Autodesk Inventor part; units mm, degrees
ref_plane "YZ Plane" through (0, 0, 0) normal (1, 0, 0) x (0, 1, 0)
ref_plane "XZ Plane" through (0, 0, 0) normal (0, 1, 0) x (-1, 0, 0)
ref_plane "XY Plane" through (0, 0, 0) normal (0, 0, 1) x (1, 0, 0)
sketch "Boceto1" plane through (0, 0, 0) normal (0, 1, 0) x (-1, 0, 0)
  line L0 (-13, -23) -> (13, -23)
  line L1 (13, -23) -> (13, 23)
  line L2 (13, 23) -> (-13, 23)
  line L3 (-13, 23) -> (-13, -23)
  line L4 (-13, -23) -> (13, 23) construction
  line L5 (13, -23) -> (-13, 23) construction
  line L6 (-14.5, -25) -> (14.5, -25)
  line L7 (14.5, -25) -> (14.5, 25)
  line L8 (14.5, 25) -> (-14.5, 25)
  line L9 (-14.5, 25) -> (-14.5, -25)
  line L10 (-14.5, -25) -> (14.5, 25) construction
  line L11 (14.5, -25) -> (-14.5, 25) construction
  point P0 (0, 0)
  dimension "d0" = 46
  dimension "d1" = 26
  dimension "d2" = 2
  dimension "d3" = 1.5
extrude "Extrusión1" add sketch "Boceto1" along normal blind 19.5 contours L3 L2 L1 L0 | L9 L8 L7 L6
sketch "Boceto2" plane through (0, 19.5, 0) normal (0, 1, 0) x (1, 0, 0)
  line L0 (-13, -23) -> (13, -23)
  line L1 (13, -23) -> (13, 23)
  line L2 (13, 23) -> (-13, 23)
  line L3 (-13, 23) -> (-13, -23)
  point P0 (0, 0)
extrude "Extrusión2" cut sketch "Boceto2" against normal blind 16.25
sketch "Boceto3" plane through (-14.5, 0, 25) normal (0, 0, 1) x (1, 0, 0)
  line L0 (29, 19.5) -> (0, 19.5)
  line L1 (13.0274, 19.5) -> (13.0274, 8.5)
  line L2 (17.0274, 19.5) -> (17.0274, 8.5)
  line L3 (3.0274, 19.5) -> (3.0274, 8.5)
  line L4 (27.0274, 19.5) -> (27.0274, 8.5)
  arc A0 (3.0274, 8.5) -> (13.0274, 8.5) centre (8.0274, 8.5) ccw
  arc A1 (17.0274, 8.5) -> (27.0274, 8.5) centre (22.0274, 8.5) ccw
  point P0 (14.5, 0)
  dimension "d8" = 11
  dimension "d10" = 10
  dimension "d11" = 10
  dimension "d12" = 4
  dimension "d13" = 11
  dimension "d14" = 11
  dimension "d15" = 11
extrude "Extrusión3" cut sketch "Boceto3" against normal blind 17
sketch "Boceto4" plane through (-14.5, 0, -25) normal (-1, 0, 0) x (0, 0, 1)
  line L0 (48, 19.5) -> (2, 19.5)
  arc A0 (10.16, 19.5) -> (39.84, 19.5) centre (25, 30.7495) ccw
  line L1 (0, 0) -> (0, 19.5)
  line L2 (50, 0) -> (50, 19.5)
  point P0 (25, 0)
  dimension "d18" = 10.16
  dimension "d19" = 10.16
extrude "Extrusión4" cut sketch "Boceto4" against normal blind 17
sketch "Boceto5" plane through (14.5, 0, 25) normal (1, 0, 0) x (0, 0, -1)
  line L0 (48, 19.5) -> (2, 19.5)
  arc A0 (10.16, 19.5) -> (39.84, 19.5) centre (25, 35.1546) ccw
  line L1 (50, 0) -> (50, 19.5)
  line L2 (0, 0) -> (0, 19.5)
  point P0 (25, 0)
  dimension "d22" = 10.16
  dimension "d23" = 10.16
extrude "Extrusión5" cut sketch "Boceto5" against normal blind 17
fillet "Empalme1" radius 2 8 edges at (13.75, 19.5, -14.84) (13.75, 19.5, 14.84) (13.5137, 19.5, 25) (-13.75, 19.5, -14.84) (-13.75, 19.5, 14.84) (-12.9863, 19.5, 25) (0.5274, 19.5, 25) (0, 19.5, -25)
properties part number "CASE batería"
The model under review builds one solid part; all positions refer to its coordinate system, in mm. A direction names the side the tool comes from. Give positions to 0.01 mm unless a question says otherwise; leave off trailing zeros. Write each loop counter-clockwise with the first axis right and the second up, starting at its lowest first coordinate (ties: lowest second). Pieces come first, ordered by that corner, then holes. Notation, with made-up numbers: (64.5, 1) - (94.5, 1) arc R21 cw to (94.5, 23) - close; hole circle Ø9 at (44.25, 2.25). An arc over 180 degrees is marked (long way). Answer in a Markdown table with one row per item. Add a question column.
1. We need section B-B on y = 18.25. Write out the cut boundary in (x, z), then the cut area to 3 significant figures.
2. Draft analysis for pull direction X (two halves, no side actions). For faces 6 (the flat face through (-11.473, 14, 24)), 7 (the flat face through (14, 19.5, 19)), state which applies: +X half, -X half, draft (parallel to the pull), parting line (faces both ways), or undercut.
3. Wall thickness on line 1 along X through (y, z) = (8, 22.5); line 2 along Z through (x, y) = (-3.5, 3.5); line 3 along Y through (x, z) = (2.75, -1): over which ranges is each line inside the solid? List them lowest first. Write a range as [from, to].
4. Tool access review of faces 1 (the flat face through (13, 10, 0)), 2 (the cylindrical face through (13.74, 19.374, 14.918)), 3 (the cylindrical face through (-13.74, 19.32, -14.97)), 4 (the flat face through (-1.473, 14, 24)), 5 (the cylindrical face through (13.53, 18.93, 24.4)): name each direction out of +Z, -Z, +X, -X, +Y, -Y from which nothing blocks a thin tool from reaching the whole face with its end or side.
5. We need section D-D on z = 0. Write out the cut boundary in (x, y), then the cut area to 3 significant figures.
6. We need section A-A on z = -17. Write out the cut boundary in (x, y).
7. Insertion check: P1, Ø8, axis at x = 3, z = -8.5, coming from the +Y side; P2, Ø6, axis at x = -8, y = 14, coming from the +Z side; P3, Ø8, axis at x = -11, z = 7.5, coming from the +Y side; P4, Ø3, axis at y = 15.5, z = -3.5, coming from the +X side. Each pin has a flat end and moves straight along its axis. Give the tip position at first contact, or say it passes through.
Ans:
| question | item | result |
|---|---|---|
| 1 | outline | (-14.5, -24.85) - (14.5, -24.85) - (14.5, -13.4) - (13, -13.4) - (13, -23) - (-13, -23) - (-13, -13.8) - (-14.5, -13.8) - close; (-14.5, 13.8) - (-13, 13.8) - (-13, 23) - (-11.47, 23) - (-11.47, 24.85) - (-14.5, 24.85) - close; (-1.47, 23) - (2.53, 23) - (2.53, 24.85) - (-1.47, 24.85) - close; (12.53, 23) - (13, 23) - (13, 13.4) - (14.5, 13.4) - (14.5, 24.85) - (12.53, 24.85) - close |
| 1 | area | 127 mm^2 |
| 2 | face 6 | undercut |
| 2 | face 7 | draft |
| 3 | line 1 | x = [-14.5, -13], [13, 14.5] |
| 3 | line 2 | z = [-25, -23], [23, 25] |
| 3 | line 3 | y = [0, 3.25] |
| 4 | face 1 | +Y |
| 4 | face 2 | +X, -X, +Y |
| 4 | face 3 | -X, +Y |
| 4 | face 4 | +Z, +Y |
| 4 | face 5 | +Z, +X, -X, +Y |
| 5 | outline | (-14.5, 0) - (14.5, 0) - (14.5, 13.58) - (13, 13.58) - (13, 3.25) - (-13, 3.25) - (-13, 12.13) - (-14.5, 12.13) - close |
| 5 | area | 123 mm^2 |
| 6 | outline | (-14.5, 0) - (14.5, 0) - (14.5, 19.5) - (13, 19.5) - (13, 3.25) - (-13, 3.25) - (-13, 19.5) - (-14.5, 19.5) - close |
| 7 | P1 | stops at y = 3.25 |
| 7 | P2 | stops at z = -23 |
| 7 | P3 | stops at y = 15.7 |
| 7 | P4 | passes through |
